Source: CAD feature listing. Evaluate the final solid. Frame: model axes, mm. Face numbers are marked on the shaded views. A direction names the side the tool comes from. Give positions to 0.01 mm unless a question says otherwise; leave off trailing zeros. Order: outer loops, then holes, each group sorted by start corner. A loop starts at its lowest first (then second) coordinate and runs counter-clockwise, first axis right, second up.
1) Material intervals for line 1 (Y direction, x = -0.5, z = 7.25); line 2 (Z direction, x = -4, y = -5); line 3 (Z direction, x = -10.5, y = 2.25), sorted ascending.
2) Draft query along Y for the marked faces 4, 5, 6 and 7. Return one class per face: released by +Y, released by -Y, zero draft, split by the parting line, or undercut.
3) First-contact query: P1, Ø1.5, axis at y = 2, z = 4.5, coming from the -X side; P2, Ø2.5, axis at x = -3.5, y = -5.5, coming from the +Z side; P3, Ø2.5, axis at y = 5.5, z = 6, coming from the +X side; P4, Ø1.8, axis at x = 1.06, z = 8, coming from the -Y side. Flat tips, straight axial feed; report the tip coordinate or a pass-through.
4) Section C-C, the plane x = 5.5. Return loops of the section in (y, z), plus the area to 3 significant figures.
5) Section A-A, the plane z = 7.5. Return loops of the section in (x, y), plus the area to 3 significant figures.
6) Access query for the marked faces 1, 2 and 3. Directions: +Z, -Z, +X, -X, +Y, -Y. A direction counts if a zero-diameter tool reaches every point of the face in a straight line with its end or side. Return the directions, or none.
7) Section B-B, the plane y = 0. Return loops of the section in (x, z), plus the area to 3 significant figures.
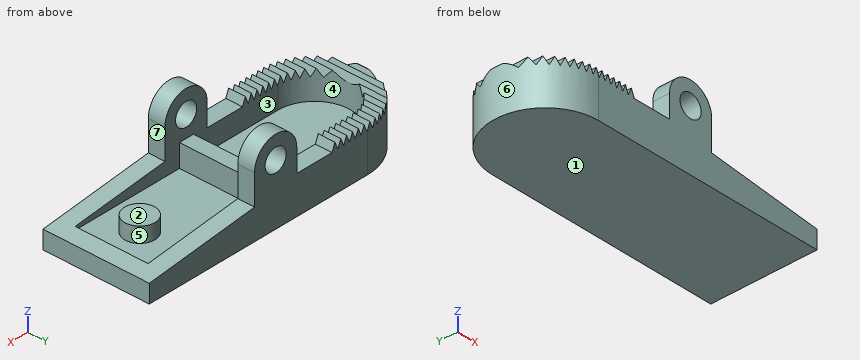
```python
from build123d import *

# Parameters (mm, degrees)
F1_DEPTH  = 25
F2_T      = -2.2
F3_R      = 1.5
F4_DEPTH  = 12.5
F5_R      = 2
F6_DEPTH  = 2
F7_W      = 2
F7_H      = 9.6
F8_DEPTH  = 3
F10_DEPTH = 14


with BuildPart() as f1:
    # F0 (on Top) → F1 (new body)
    with BuildSketch(Plane.XY):
        with BuildLine():
            Line((19, 7), (-12, 7))
            ThreePointArc((-12, 7), (-19, 0), (-12, -7))
            Line((-12, -7), (19, -7))
            Line((19, -7), (19, 7))
        make_face()
    extrude(amount=F1_DEPTH)

    # F2
    f2_openings = [f1.faces().sort_by_distance(p)[0] for p in [
        (0.717666, 0, 25),
    ]]
    offset(amount=F2_T, openings=f2_openings)

    # F3 (on Front) → F4 (cut, symmetric)
    with BuildSketch(Plane.XZ):
        with BuildLine():
            Line((4.05511, 8), (4.05511, 4))
            Line((4.05511, 4), (19, 2.4))
            Line((19, 2.4), (19, 25))
            Line((19, 25), (-19.30074, 25))
            Line((-19.30074, 25), (-19.30074, 6))
            Line((-19.30074, 6), (-6.94489, 6))
            Line((-6.94489, 6), (-6.94489, 5))
            Line((-6.94489, 5), (-1.94489, 5))
            Line((-1.94489, 5), (-1.94489, 8))
            ThreePointArc((-1.94489, 8), (1.05511, 11), (4.05511, 8))
        make_face()
        with Locations((1.05511, 8)):
            Circle(F3_R)
    extrude(amount=F4_DEPTH, both=True, mode=Mode.SUBTRACT)

    # F5 (on face) → F6 (join)
    with BuildSketch(Plane.XY.offset(2.2)):
        with Locations((12.8, 0)):
            Circle(F5_R)
    extrude(amount=F6_DEPTH)

    # F7 (on face) → F8 (join)
    with BuildSketch(Plane.XY.offset(2.2)):
        with Locations((1, 0)):
            Rectangle(F7_W, F7_H)
    extrude(amount=F8_DEPTH)

    # F9 (on face) → F10 (cut, through all)
    with BuildSketch(Plane.XZ.offset(7)):
        Polygon((-18.54287, 5), (-18.128656, 6), (-18.957083, 6), align=None)
        Polygon((-17.714443, 5), (-17.300229, 6), (-18.128656, 6), align=None)
        Polygon((-16.886015, 5), (-16.471802, 6), (-17.300229, 6), align=None)
        Polygon((-16.057588, 5), (-15.643375, 6), (-16.471802, 6), align=None)
        Polygon((-15.229161, 5), (-14.814948, 6), (-15.643375, 6), align=None)
        Polygon((-14.400734, 5), (-13.98652, 6), (-14.814948, 6), align=None)
        Polygon((-13.572307, 5), (-13.158093, 6), (-13.98652, 6), align=None)
        Polygon((-12.74388, 5), (-12.329666, 6), (-13.158093, 6), align=None)
        Polygon((-11.915453, 5), (-11.501239, 6), (-12.329666, 6), align=None)
        Polygon((-11.087026, 5), (-10.672812, 6), (-11.501239, 6), align=None)
        Polygon((-10.258598, 5), (-9.844385, 6), (-10.672812, 6), align=None)
        Polygon((-9.430171, 5), (-9.015958, 6), (-9.844385, 6), align=None)
        Polygon((-8.601744, 5), (-8.187531, 6), (-9.015958, 6), align=None)
        Polygon((-7.773317, 5), (-7.359103, 6), (-8.187531, 6), align=None)
        Polygon((-6.94489, 5), (-6.530676, 6), (-7.359103, 6), align=None)
    extrude(amount=-F10_DEPTH, mode=Mode.SUBTRACT)


solid = f1.part
```
From the geometry:
1. line 1: y = -7 to -4.8, 4.8 to 7
1. line 2: z = 0 to 5
1. line 3: z = 0 to 2.2
2. face 4: undercut
2. face 5: undercut
2. face 6: split by the parting line
2. face 7: zero draft
3. P1: stops at x = -18.89
3. P2: stops at z = 5
3. P3: stops at x = 4.06
3. P4: passes through
4. outline: (-7, 0) - (7, 0) - (7, 3.85) - (4.8, 3.85) - (4.8, 2.2) - (-4.8, 2.2) - (-4.8, 3.85) - (-7, 3.85) - close
4. area: 38.0 mm2
5. outline: (-1.94, -7) - (-0.36, -7) - (-0.36, -4.8) - (-1.94, -4.8) - close; (-1.94, 4.8) - (-0.36, 4.8) - (-0.36, 7) - (-1.94, 7) - close; (2.47, -7) - (4.06, -7) - (4.06, -4.8) - (2.47, -4.8) - close; (2.47, 4.8) - (4.06, 4.8) - (4.06, 7) - (2.47, 7) - close
5. area: 14.0 mm2
6. face 1: -Z, +X, -X, +Y, -Y
6. face 2: +Z, +X, +Y, -Y
6. face 3: +Z
7. outline: (-19, 0) - (19, 0) - (19, 2.4) - (16.8, 2.64) - (16.8, 2.2) - (14.8, 2.2) - (14.8, 4.2) - (10.8, 4.2) - (10.8, 2.2) - (2, 2.2) - (2, 5.2) - (0, 5.2) - (0, 2.2) - (-16.8, 2.2) - (-16.8, 5.21) - (-16.89, 5) - (-17.3, 6) - (-17.71, 5) - (-18.13, 6) - (-18.54, 5) - (-18.96, 6) - (-19, 6) - close
7. area: 106 mm2
